from build123d import *

# Parameters (mm, degrees)
SZKIC1_W                    = 200
SZKIC1_H                    = 250
DODANIE_WYCI_GNI_CIE1_DEPTH = 3
SZKIC2_R                    = 2.1
SZKIC2_R_2                  = 3.1
WYTNIJ_WYCI_GNI_CIE1_DEPTH  = 321.170267202


with BuildPart() as part:
    # Szkic1 → Dodanie-wyciągnięcie1 (new body)
    with BuildSketch(Plane.XY):
        with Locations((100, 125)):
            Rectangle(SZKIC1_W, SZKIC1_H)
    extrude(amount=DODANIE_WYCI_GNI_CIE1_DEPTH)

    # Szkic2 → Wytnij-wyciągnięcie1 (cut, through all)
    with BuildSketch(Plane.XY.offset(3)):
        with Locations((18.2, 165)):
            Circle(SZKIC2_R)
        with Locations((56.4, 231.8)):
            Circle(SZKIC2_R_2)
        with Locations((143.6, 231.8)):
            Circle(SZKIC2_R_2)
        with Locations((167.8, 205)):
            Circle(SZKIC2_R)
        with Locations((181.8, 205)):
            Circle(SZKIC2_R)
        with Locations((18.2, 205)):
            Circle(SZKIC2_R)
        with Locations((32.2, 205)):
            Circle(SZKIC2_R)
        with Locations(Location((181.8, 165, 0), (0, 0, 180))):
            Circle(SZKIC2_R)
    extrude(amount=-WYTNIJ_WYCI_GNI_CIE1_DEPTH, mode=Mode.SUBTRACT)


solid = part.part
Here's how the part is built. I have some questions about the finished solid (model axes, mm). Round coordinates to 2 decimals unless told otherwise and drop trailing zeros. Loops run counter-clockwise (first coordinate to the right, second up) from the corner with the lowest first, then second, coordinate; pieces in that order, holes last. Notation, with made-up numbers: (88.5, 83) -> (146.5, 83) arc R29 cw to (146.5, 111) -> close; hole circle Ø6 at (39, 59). An arc over 180 degrees is marked (long way). Write each question's results on one line, items separated by ' | '.
(1) We'd pull the mould along Y, two halves only. Please class faces 1 (the face through (99, 127, 0)), 2 (the face through (146.557, 232.731, 1.521)), 3 (the face through (55.996, 234.874, 1.521)): released by +Y, released by -Y, zero draft, split by the parting line, or undercut.
Worked answers:
face 1: zero draft | face 2: undercut | face 3: undercut
(2) For P1, Ø2.5, axis at x = 181.8, y = 205, coming from the -Z side, with a flat end and sliding along its axis, tell me the tip position at first contact or that it passes through.
Worked answers:
P1: through
(3) If we section it at B-B, the plane y = 231.8: List the corners of the cut face in (x, z) for me, then the cut area to 3 significant figures.
Worked answers:
outline: (0, 0) -> (53.3, 0) -> (53.3, 3) -> (0, 3) -> close; (59.5, 0) -> (140.5, 0) -> (140.5, 3) -> (59.5, 3) -> close; (146.7, 0) -> (200, 0) -> (200, 3) -> (146.7, 3) -> close | area: 563 mm2
(4) If I drill on L1, parallel to Y at x = 181.8, z = 1.35; L2, parallel to X at y = 205, z = 2.2; L3, parallel to X at y = 231.8, z = 1.6, over which ranges is the centre line in solid material (lowest first)?
Worked answers:
L1: 0 to 162.9, 167.1 to 202.9, 207.1 to 250 | L2: 0 to 16.1, 20.3 to 30.1, 34.3 to 165.7, 169.9 to 179.7, 183.9 to 200 | L3: 0 to 53.3, 59.5 to 140.5, 146.7 to 200
(5) If we section it at A-A, the plane x = 143.6: List the corners of the cut face in (y, z) for me, then the cut area to 3 significant figures.
Worked answers:
outline: (0, 0) -> (228.7, 0) -> (228.7, 3) -> (0, 3) -> close; (234.9, 0) -> (250, 0) -> (250, 3) -> (234.9, 3) -> close | area: 731 mm2
